For this review, take the finished solid that the model builds, in its own axes (mm). A direction names the side the tool comes from. Round coordinates to 2 decimals unless told otherwise and drop trailing zeros. Loops run counter-clockwise (first coordinate to the right, second up) from the corner with the lowest first, then second, coordinate; pieces in that order, holes last. Notation, with made-up numbers: (34, 43.5) -> (73, 43.5) arc R16 cw to (73, 71.5) -> close; hole circle Ø4 at (-11.5, 20). An arc over 180 degrees is marked (long way). One line per question, with ' | ' between items. Start each with the question number.
1. Consider section B-B (x = 8.5). Write out the cut boundary in (y, z) (3 decimals).
2. Consider section D-D (z = 2.75). Write out the cut boundary in (x, y).
3. For pin 1 Ø5 at (x, z) = (-25, -3.5) entering from +Y; pin 2 Ø2.5 at (x, y) = (0, 20.955) entering from +Z (3 decimals); pin 3 Ø4 at (x, z) = (-26, -7) entering from -Y; pin 4 Ø2.5 at (x, y) = (-26.04, -26.04) entering from -Z, all flat-tipped, find the tip position at first contact; note any pin that passes through.
4. Consider section C-C (z = -6.5). Write out the cut boundary in (x, y), and give its area (3 significant figures).
5. For faces 4 (the face through (24.486, 26.533, 1.878)), 5 (the face through (-16, 7, -0.838)), list the 3-axis set-ups (+Z, -Z, +X, -X, +Y, -Y) from which the entire face can be reached by the end or side of a thin tool; tool diameter is ignored.
6. Consider section A-A (y = 0). Write out the cut boundary in (x, z) (3 decimals), and give its area (3 significant figures).
7. Draft analysis for pull direction X (two halves, no side actions). For faces 1 (the face through (23.016, 7.248, 2.245)), 2 (the face through (-10, -27, 0)), 3 (the face through (3.64, 27.7, -4.38)), state which applies: pulls with the +X half, pulls with the -X half, needs draft (parallel to the pull), parting line crosses it, or undercut.
8. Wall thickness on line 1 along X through (y, z) = (-1, 0.25); line 2 along Z through (x, y) = (12, 30); line 3 along Z through (x, y) = (-12.5, 11) (3 decimals): over which ranges is each line inside the solid? List them lowest first.
```python
from build123d import *

# Parameters (mm, degrees)
SKETCH1_R             = 40.64
EXTRUDE1_DEPTH        = 3.81
F_4_CLEARANCE_HOLE1_D = 3.2639
SKETCH6_R             = 27.94
EXTRUDE2_DEPTH        = 8.89
SKETCH5_R             = 16.51
CUT_EXTRUDE2_DEPTH    = 13.7
SKETCH14_R            = 24.13
CUT_EXTRUDE3_DEPTH    = 3.175
CIRPATTERN1_COUNT     = 3
SKETCH13_R            = 19.177
SKETCH13_R_2          = 17.2593
CUT_EXTRUDE4_DEPTH    = 1.4732


with BuildPart() as part:
    # Sketch1 → Extrude1 (new body)
    with BuildSketch(Plane.XY):
        Circle(SKETCH1_R)
    extrude(amount=EXTRUDE1_DEPTH)

    # #4 Clearance Hole1 (through all)
    with Locations(Plane.XY.offset(3.81)):
        with Locations((26.042742751, 26.042742751), (26.042742751, -26.042742751), (-26.042288216, 26.043197279), (-26.04251548, -26.04297002)):
            Hole(F_4_CLEARANCE_HOLE1_D / 2)

    # Sketch6 → Extrude2 (add)
    with BuildSketch(Plane(origin=(0, 0, 0), x_dir=(-1, 0, 0), z_dir=(0, 0, -1))):
        Circle(SKETCH6_R)
    extrude(amount=EXTRUDE2_DEPTH)

    # Sketch5 → Cut-Extrude2 (cut, through all)
    with BuildSketch(Plane.XY.offset(3.81)):
        Circle(SKETCH5_R)
    extrude(amount=-CUT_EXTRUDE2_DEPTH, mode=Mode.SUBTRACT)

    # Sketch14 → Cut-Extrude3 (cut)
    with BuildSketch(Plane.XY.offset(3.81)):
        Circle(SKETCH14_R)
    extrude(amount=-CUT_EXTRUDE3_DEPTH, mode=Mode.SUBTRACT)

    # Sketch16 → #2-56 Tapped Hole1 (revolve, cut)
    with BuildSketch(Plane(origin=(0, 20.955, 0.635), x_dir=(0, -1, 0), z_dir=(1, 0, 0))):
        Polygon((0, 0), (0, 4.95376509), (0.889, 4.4196), (0.889, 0), align=None)
    f_2_56_tapped_hole1 = revolve(axis=Axis((0, 20.955, 6.985), (0, 0, -1)), mode=Mode.SUBTRACT)

    # CirPattern1: #2-56 Tapped Hole1 ×3 about axis
    cirpattern1_axis = Axis((0, 0, 0), (0, 0, 1))
    for i in range(1, CIRPATTERN1_COUNT):
        add(f_2_56_tapped_hole1.rotate(cirpattern1_axis, i * 360 / CIRPATTERN1_COUNT), mode=Mode.SUBTRACT)

    # Sketch13 → Cut-Extrude4 (cut)
    with BuildSketch(Plane.XY.offset(0.635)):
        Circle(SKETCH13_R)
        Circle(SKETCH13_R_2, mode=Mode.SUBTRACT)
    extrude(amount=-CUT_EXTRUDE4_DEPTH, mode=Mode.SUBTRACT)


solid = part.part
```
Answer block:
1) outline: (-39.741, 0) -> (-26.616, 0) -> (-26.616, -8.89) -> (-14.154, -8.89) -> (-14.154, 0.635) -> (-15.021, 0.635) -> (-15.021, -0.838) -> (-17.19, -0.838) -> (-17.19, 0.635) -> (-22.583, 0.635) -> (-22.583, 3.81) -> (-39.741, 3.81) -> close; (14.154, -8.89) -> (26.616, -8.89) -> (26.616, 0) -> (39.741, 0) -> (39.741, 3.81) -> (22.583, 3.81) -> (22.583, 0.635) -> (17.19, 0.635) -> (17.19, -0.838) -> (15.021, -0.838) -> (15.021, 0.635) -> (14.154, 0.635) -> close
2) outline: circle Ø81.28 at (0, 0); hole circle Ø3.26 at (-26.04, -26.04); hole circle Ø3.26 at (-26.04, 26.04); hole circle Ø48.26 at (0, 0); hole circle Ø3.26 at (26.04, -26.04); hole circle Ø3.26 at (26.04, 26.04)
3) pin 1: stops at y = 16.56 | pin 2: stops at z = 0.635 | pin 3: stops at y = -14.31 | pin 4: passes through
4) outline: circle Ø55.88 at (0, 0); hole circle Ø33.02 at (0, 0) | area: 1,600 mm2
5) face 4: +Z, -Z | face 5: +Z
6) outline: (-40.64, 0) -> (-27.94, 0) -> (-27.94, -8.89) -> (-16.51, -8.89) -> (-16.51, 0.635) -> (-17.259, 0.635) -> (-17.259, -0.838) -> (-19.177, -0.838) -> (-19.177, 0.635) -> (-24.13, 0.635) -> (-24.13, 3.81) -> (-40.64, 3.81) -> close; (16.51, -8.89) -> (27.94, -8.89) -> (27.94, 0) -> (40.64, 0) -> (40.64, 3.81) -> (24.13, 3.81) -> (24.13, 0.635) -> (19.177, 0.635) -> (19.177, -0.838) -> (17.259, -0.838) -> (17.259, 0.635) -> (16.51, 0.635) -> close | area: 333 mm2
7) face 1: undercut | face 2: needs draft | face 3: parting line crosses it
8) line 1: x = -40.63 to -19.15, -17.23 to -16.48, 16.48 to 17.23, 19.15 to 40.63 | line 2: z = 0 to 3.81 | line 3: z = -8.89 to 0.635
